Job drawing, mm, ordinate dimensions from the low corner. One solid piece. Give positions to 0.01 mm unless a question says otherwise; leave off trailing zeros. Loops run counter-clockwise (first coordinate to the right, second up) from the corner with the lowest first, then second, coordinate; pieces in that order, holes last. Notation, with made-up numbers: M 27.5,13.25 L 84.5,13.25 A22 cw 84.5,27.25 Z; hole C 60,79 d9. An arc over 180 degrees is marked long. Put each result on its own line as item: value.
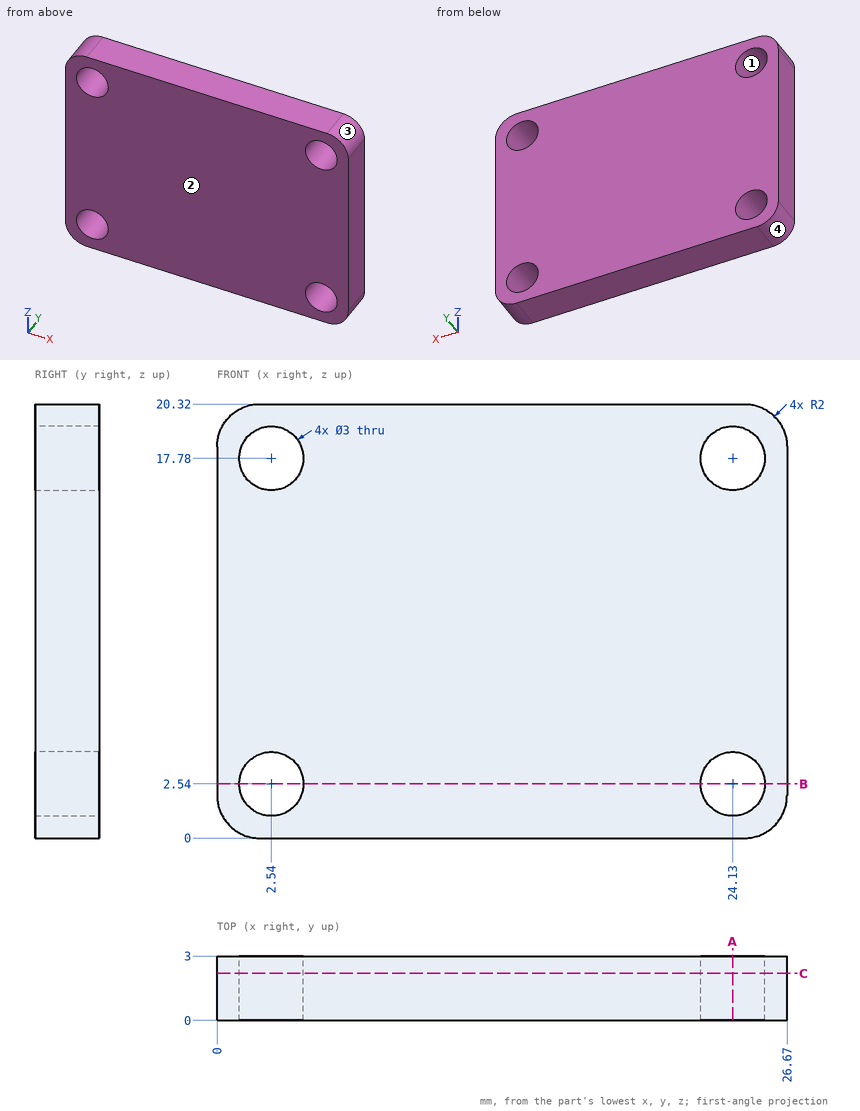
Q1. Drop a flat-ended pin along its axis: pin 1 Ø1.8 at (x, z) = (24.13, 2.54) entering from -Y. Give the stop position or say it passes through.
Here are the results:
pin 1: through
Q2. Mould opens along Z. For the marked faces 1, 2, 3 and 4 say: pulls with the +Z half, pulls with the -Z half, needs draft (parallel to the pull), parting line crosses it, or undercut.
Here are the results:
face 1: undercut
face 2: needs draft
face 3: pulls with the +Z half
face 4: pulls with the -Z half
Q3. Slice it at C-C (y = 2.2). List the corners of the cut face in (x, z).
Here are the results:
outline: M 0,2 A2 ccw 2,0 L 24.67,0 A2 ccw 26.67,2 L 26.67,18.32 A2 ccw 24.67,20.32 L 2,20.32 A2 ccw 0,18.32 Z; hole C 2.54,2.54 d3; hole C 2.54,17.78 d3; hole C 24.13,2.54 d3; hole C 24.13,17.78 d3
Q4. Slice it at B-B (z = 2.54). List the corners of the cut face in (x, y), and give its area (3 significant figures).
Here are the results:
outline: M 0,0 L 1.04,0 L 1.04,3 L 0,3 Z; M 4.04,0 L 22.63,0 L 22.63,3 L 4.04,3 Z; M 25.63,0 L 26.67,0 L 26.67,3 L 25.63,3 Z
area: 62.0 mm²
Q5. Slice it at A-A (x = 24.13). List the corners of the cut face in (y, z), and give its area (3 significant figures).
Here are the results:
outline: M 0,0 L 3,0 L 3,1.04 L 0,1.04 Z; M 0,4.04 L 3,4.04 L 3,16.28 L 0,16.28 Z; M 0,19.28 L 3,19.28 L 3,20.32 L 0,20.32 Z
area: 43.0 mm²
Q6. Probe line 1 (X direction, y = 2.15, z = 2.54); line 2 (X direction, y = 1.5, z = 1.25); line 3 (Z direction, x = 1.5, y = 1.7). List the from-to ranges inside material, lowest first. Write a range as from..to.
Here are the results:
line 1: 0..1.04, 4.04..22.63, 25.63..26.67
line 2: 0.15..1.77, 3.31..23.36, 24.9..26.52
line 3: 0.06..1.46, 3.62..16.7, 18.86..20.26
